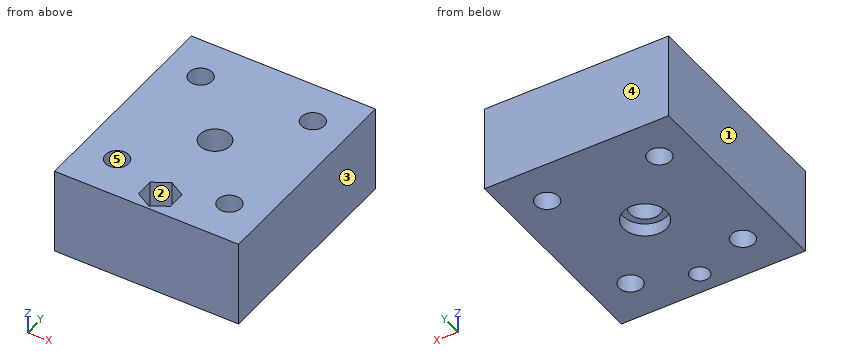
from build123d import *

# Parameters (mm, degrees)
SKETCH1_W           = 42.62295082
SKETCH1_H           = 50
SKETCH1_R           = 2.677018134
BOSS_EXTRUDE1_DEPTH = 20
SKETCH2_R           = 5.025
CUT_EXTRUDE2_DEPTH  = 3
SKETCH3_R           = 2.2
CUT_EXTRUDE3_DEPTH  = 10
CUT_EXTRUDE4_START  = -7
CUT_EXTRUDE4_DEPTH  = 32.460095998
SKETCH6_R           = 3.5
CUT_EXTRUDE5_DEPTH  = 39.460095998


with BuildPart() as part:
    # Sketch1 → Boss-Extrude1 (new body)
    with BuildSketch(Plane.XY):
        Rectangle(SKETCH1_W, SKETCH1_H)
        with Locations((-13, -15.25)):
            Circle(SKETCH1_R, mode=Mode.SUBTRACT)
        with Locations(Location((13, -15.25, 0), (0, 0, 180))):
            Circle(SKETCH1_R, mode=Mode.SUBTRACT)
        with Locations((13, 15.25)):
            Circle(SKETCH1_R, mode=Mode.SUBTRACT)
        with Locations(Location((-13, 15.25, 0), (0, 0, 180))):
            Circle(SKETCH1_R, mode=Mode.SUBTRACT)
    extrude(amount=BOSS_EXTRUDE1_DEPTH)

    # Sketch2 → Cut-Extrude2 (cut)
    with BuildSketch(Plane.XY):
        Circle(SKETCH2_R)
    extrude(amount=CUT_EXTRUDE2_DEPTH, mode=Mode.SUBTRACT)

    # Sketch3 → Cut-Extrude3 (cut)
    with BuildSketch(Plane(origin=(0, 0, 0), x_dir=(-1, 0, 0), z_dir=(0, 0, -1))):
        with Locations((0, -20)):
            Circle(SKETCH3_R)
    extrude(amount=-CUT_EXTRUDE3_DEPTH, mode=Mode.SUBTRACT)

    # Sketch5 → Cut-Extrude4 (cut, through all)
    with BuildSketch(Plane(origin=(0, 0, 0), x_dir=(-1, 0, 0), z_dir=(0, 0, -1)).offset(CUT_EXTRUDE4_START)):
        Polygon((0, -15.727608008), (-3.7, -17.863804004), (-3.7, -22.136195996), (0, -24.272391992), (3.7, -22.136195996), (3.7, -17.863804004), align=None)
    extrude(amount=-CUT_EXTRUDE4_DEPTH, mode=Mode.SUBTRACT)

    # Sketch6 → Cut-Extrude5 (cut, through all)
    with BuildSketch(Plane.XY):
        Circle(SKETCH6_R)
    extrude(amount=CUT_EXTRUDE5_DEPTH, mode=Mode.SUBTRACT)


solid = part.part
Design review of the part built by this model. Coordinates are the model's own, in mm. Face numbers are marked on the shaded views. A direction names the side the tool comes from. Coordinates: 2 decimals unless noted, no trailing zeros. Order: outer loops, then holes, each group sorted by start corner. A loop starts at its lowest first (then second) coordinate and runs counter-clockwise, first axis right, second up. Notation, with made-up numbers: (32, 18) -> (87, 18) arc R23 ccw to (87, 41) -> close; hole circle Ø6 at (38, -10). An arc over 180 degrees is marked (long way). Use one line per item in the form item = value. Start each with the question number.
(1) Insertion check: pin 1 (5 mm diameter, centred on x = -1.5, y = -1.5, fed in from -Z); pin 2 (6 mm diameter, centred on x = 0, y = 0, fed in from +Z). Each pin has a flat end and moves straight along its axis. Give the tip position at first contact, or say it passes through.
(2) Add section A-A on y = 0. State the section outline as (x, z) points (3 decimals).
(3) For probe 1 along Y at (x, z) = (13, 10.25); probe 2 along Y at (x, z) = (0, 4); probe 3 along X at (y, z) = (-21.5, 14.25), list the stretches that pass through material, from the lowest coordinate up.
(4) The part is to be moulded in two halves that separate along X. For the marked faces 3, 4 and 5, say which applies: +X half, -X half, draft (parallel to the pull), parting line (faces both ways), or undercut.
(5) For the marked faces 1 and 2, list the 3-axis set-ups (+Z, -Z, +X, -X, +Y, -Y) from which the entire face can be reached by the end or side of a thin tool; tool diameter is ignored.
(6) Add section B-B on x = -13. State the section outline as (y, z) points.
(7) Add section D-D on z = 12.25. State the section outline as (x, y) points, plus the area to 3 significant figures.
(8) Add section C-C on y = 15.25. State the section outline as (x, z) points.
Answer block:
q1.pin_1 = 3
q1.pin_2 = through
q2.outline = (-21.311, 0) -> (-5.025, 0) -> (-5.025, 3) -> (-3.5, 3) -> (-3.5, 20) -> (-21.311, 20) -> close; (3.5, 3) -> (5.025, 3) -> (5.025, 0) -> (21.311, 0) -> (21.311, 20) -> (3.5, 20) -> close
q3.probe_1 = -25 to -17.93, -12.57 to 12.57, 17.93 to 25
q3.probe_2 = -25 to -22.2, -17.8 to -3.5, 3.5 to 25
q3.probe_3 = -21.31 to -3.7, 3.7 to 21.31
q4.face_3 = +X half
q4.face_4 = draft
q4.face_5 = undercut
q5.face_1 = +Z, -Z, -X, +Y, -Y
q5.face_2 = +Z
q6.outline = (-25, 0) -> (-17.93, 0) -> (-17.93, 20) -> (-25, 20) -> close; (-12.57, 0) -> (12.57, 0) -> (12.57, 20) -> (-12.57, 20) -> close; (17.93, 0) -> (25, 0) -> (25, 20) -> (17.93, 20) -> close
q7.outline = (-21.31, -25) -> (21.31, -25) -> (21.31, 25) -> (-21.31, 25) -> close; hole circle Ø5.35 at (-13, -15.25); hole circle Ø5.35 at (-13, 15.25); hole (-3.7, -22.14) -> (0, -24.27) -> (3.7, -22.14) -> (3.7, -17.86) -> (0, -15.73) -> (-3.7, -17.86) -> close; hole circle Ø7 at (0, 0); hole circle Ø5.35 at (13, -15.25); hole circle Ø5.35 at (13, 15.25)
q7.area = 1,960 mm²
q8.outline = (-21.31, 0) -> (-15.68, 0) -> (-15.68, 20) -> (-21.31, 20) -> close; (-10.32, 0) -> (10.32, 0) -> (10.32, 20) -> (-10.32, 20) -> close; (15.68, 0) -> (21.31, 0) -> (21.31, 20) -> (15.68, 20) -> close
